```python
from build123d import *

# Parameters (mm, degrees)
F2_DEPTH     = 4
F0_R         = 11.5
F3_DEPTH     = 4
F4_T1_DEPTH  = 21.9483713996
F4_T3_DEPTH  = 22.3459559115
F4_T5_DEPTH  = 21.2495705846
F4_T7_DEPTH  = 22.5954800676
F4_T9_DEPTH  = 22.5954384353
F4_T11_DEPTH = 21.948545213


# Not quite as in the source:
# - a fillet or chamfer that OpenCascade refuses, or shapes differently, is made with other operations: its cross-section is extruded or revolved along the edge and cut away or added


with BuildPart() as f2:
    # F1 (on Top) → F2 (new body, symmetric)
    with BuildSketch(Plane.XY):
        with BuildLine():
            ThreePointArc((-24.434154737, 1.9297075548), (-16.0117202716, 5.9282775779), (-12.5894382026, 14.6008752276))
            ThreePointArc((-12.5894382026, 14.6008752276), (-12.8847624083, 17.3237447508), (-13.7570001617, 19.9199797418))
            Line((-13.7570001617, 19.9199797418), (-24.434154737, 1.9297075548))
        make_face()
        with BuildLine():
            ThreePointArc((-13.7570001617, 19.9199797418), (-12.8847624083, 17.3237447508), (-12.5894382026, 14.6008752276))
            ThreePointArc((-12.5894382026, 14.6008752276), (-16.0117202716, 5.9282775779), (-24.434154737, 1.9297075548))
            Line((-24.434154737, 1.9297075548), (-25.3981637022, 0.3054186533))
            Line((-25.3981637022, 0.3054186533), (-12.9635821636, -21.842745649))
            Line((-12.9635821636, -21.842745649), (-10.3728090059, -21.8739002812))
            ThreePointArc((-10.3728090059, -21.8739002812), (0.1527093266, -16.5024942777), (10.54601793, -22.1254538984))
            Line((10.54601793, -22.1254538984), (12.4345815386, -22.1481643023))
            Line((12.4345815386, -22.1481643023), (25.3981637022, -0.3054186533))
            Line((25.3981637022, -0.3054186533), (24.3123835544, 1.6285456733))
            ThreePointArc((24.3123835544, 1.6285456733), (13.9458157922, 8.2323089444), (13.7055148895, 20.5212337137))
            Line((13.7055148895, 20.5212337137), (12.9635821636, 21.842745649))
            Line((12.9635821636, 21.842745649), (-12.4345815386, 22.1481643023))
            Line((-12.4345815386, 22.1481643023), (-13.7570001617, 19.9199797418))
        make_face()
        with BuildLine():
            Line((-24.434154737, 1.9297075548), (-13.7570001617, 19.9199797418))
            ThreePointArc((-13.7570001617, 19.9199797418), (-36.2108110271, 21.0826663094), (-24.434154737, 1.9297075548))
        make_face()
        with BuildLine():
            Line((24.3123835544, 1.6285456733), (13.7055148895, 20.5212337137))
            ThreePointArc((13.7055148895, 20.5212337137), (13.9458157922, 8.2323089444), (24.3123835544, 1.6285456733))
        make_face()
        with BuildLine():
            ThreePointArc((38.29859269, 14.6009373546), (28.3341688507, 27.2487571734), (13.7055148895, 20.5212337137))
            Line((13.7055148895, 20.5212337137), (24.3123835544, 1.6285456733))
            ThreePointArc((24.3123835544, 1.6285456733), (34.136115438, 5.0628952085), (38.29859269, 14.6009373546))
        make_face()
        with BuildLine():
            Line((10.54601793, -22.1254538984), (-10.3728090059, -21.8739002812))
            ThreePointArc((-10.3728090059, -21.8739002812), (-3.8441725784, -41.3058041995), (12.7, -29.2015761288))
            ThreePointArc((12.7, -29.2015761288), (12.1495766945, -25.5032270182), (10.54601793, -22.1254538984))
        make_face()
        with BuildLine():
            ThreePointArc((10.54601793, -22.1254538984), (0.1527093266, -16.5024942777), (-10.3728090059, -21.8739002812))
            Line((-10.3728090059, -21.8739002812), (10.54601793, -22.1254538984))
        make_face()
    extrude(amount=F2_DEPTH, both=True)

    # F0 (on Top) → F3 (cut, symmetric)
    with BuildSketch(Plane.XY):
        with Locations((-25.4, 14.6646968374)):
            Circle(F0_R)
        with Locations((25.4, 14.6646968374)):
            Circle(F0_R)
        with Locations((0, -29.3293936748)):
            Circle(F0_R)
        Circle(F0_R)
    extrude(amount=F3_DEPTH, both=True, mode=Mode.SUBTRACT)

    # F4: fillet of radius 5.08 on 6 edges, made by hand

    # F4_s2 → F4_t1 (cut)
    with BuildSketch(Plane.XY.offset(-10.9741856998)):
        with BuildLine():
            ThreePointArc((10.54601793, -22.1254538984), (12.4510077343, -21.2841478503), (13.8583678275, -19.7491821865))
            Line((13.8583678275, -19.7491821865), (12.4345815386, -22.1481643023))
            Line((12.4345815386, -22.1481643023), (10.54601793, -22.1254538984))
        make_face()
    extrude(amount=F4_T1_DEPTH, mode=Mode.SUBTRACT)

    # F4_s4 → F4_t3 (cut)
    with BuildSketch(Plane.XY.offset(-11.1729779558)):
        with BuildLine():
            ThreePointArc((23.9337937954, -2.7727813782), (24.6265549669, -0.6154246052), (24.3123835544, 1.6285456733))
            Line((24.3123835544, 1.6285456733), (25.3981637022, -0.3054186533))
            Line((25.3981637022, -0.3054186533), (23.9337937954, -2.7727813782))
        make_face()
    extrude(amount=F4_T3_DEPTH, mode=Mode.SUBTRACT)

    # F4_s6 → F4_t5 (cut)
    with BuildSketch(Plane.XY.offset(-10.6247852923)):
        with BuildLine():
            ThreePointArc((10.3138596228, 21.8746091608), (12.1354983401, 21.5132129748), (13.7055148895, 20.5212337137))
            Line((13.7055148895, 20.5212337137), (12.9635821636, 21.842745649))
            Line((12.9635821636, 21.842745649), (10.3138596228, 21.8746091608))
        make_face()
    extrude(amount=F4_T5_DEPTH, mode=Mode.SUBTRACT)

    # F4_s8 → F4_t7 (cut)
    with BuildSketch(Plane.XY.offset(-11.2977400338)):
        with BuildLine():
            ThreePointArc((-13.7570001617, 19.9199797418), (-11.910066672, 21.54587795), (-9.5156965617, 22.1130640513))
            Line((-9.5156965617, 22.1130640513), (-12.4345815386, 22.1481643023))
            Line((-12.4345815386, 22.1481643023), (-13.7570001617, 19.9199797418))
        make_face()
    extrude(amount=F4_T7_DEPTH, mode=Mode.SUBTRACT)

    # F4_s10 → F4_t9 (cut)
    with BuildSketch(Plane.XY.offset(-11.2977192176)):
        with BuildLine():
            ThreePointArc((-14.3926228669, -19.2973742433), (-12.7042844419, -21.0873382025), (-10.3728090059, -21.8739002812))
            Line((-10.3728090059, -21.8739002812), (-12.9635821636, -21.842745649))
            Line((-12.9635821636, -21.842745649), (-14.3926228669, -19.2973742433))
        make_face()
    extrude(amount=F4_T9_DEPTH, mode=Mode.SUBTRACT)

    # F4_s12 → F4_t11 (cut)
    with BuildSketch(Plane.XY.offset(-10.9742726065)):
        with BuildLine():
            ThreePointArc((-24.0324603731, -2.1271378125), (-24.6581063385, -0.1407771898), (-24.434154737, 1.9297075548))
            Line((-24.434154737, 1.9297075548), (-25.3981637022, 0.3054186533))
            Line((-25.3981637022, 0.3054186533), (-24.0324603731, -2.1271378125))
        make_face()
    extrude(amount=F4_T11_DEPTH, mode=Mode.SUBTRACT)


solid = f2.part
```
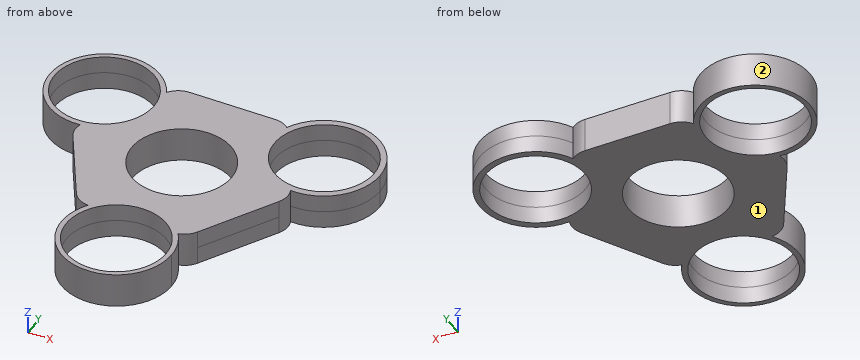
CAD build for the part. Positions are in the model's coordinates, mm. Face numbers are marked on the shaded views. Round coordinates to 2 decimals unless told otherwise and drop trailing zeros. Order: outer loops, then holes, each group sorted by start corner. A loop starts at its lowest first (then second) coordinate and runs counter-clockwise, first axis right, second up. Notation, with made-up numbers: (79, 60) - (115, 60) arc R22 cw to (115, 97) - close; hole circle Ø2 at (77, 52). An arc over 180 degrees is marked (long way). Use CSV: the item, a comma, the result in double quotes. Start each with the question number.
1) Wall check: L1, parallel to X at y = -29, z = -2.5; L2, parallel to Y at x = 25.4, z = -3.05; L3, parallel to Y at x = -25.4, z = 2.5. Give the ranges that are in metal, low to high. Write a range as [from, to].
2) Saw through at D-D (y = -31). List the corners of the cut face in (x, z).
3) Pin check, flat tips, straight feed: pin 1 Ø14 at (x, y) = (0, -29.33) entering from -Z; pin 2 Ø1.5 at (x, z) = (10, -1.5) entering from -Y. Stop position of each tip, or through.
4) Two-plate mould, pull along X, no slides. Class the marked faces 1 and 2: pulls with the +X half, pulls with the -X half, needs draft (parallel to the pull), parting line crosses it, or undercut.
5) Saw through at B-B (y = 16). List the corners of the cut face in (x, z), and give its area (3 significant figures).
6) Saw through at A-A (x = -4.5). List the corners of the cut face in (y, z).
7) Saw through at C-C (x = 19). List the corners of the cut face in (y, z), and give its area (3 significant figures).
Values follow:
1,L1,"x = [-12.7, -11.5], [11.5, 12.7]"
1,L2,"y = [1.59, 3.16], [26.16, 27.61]"
1,L3,"y = [1.9, 3.16], [26.16, 27.3]"
2,outline,"(-12.57, -4) - (-11.38, -4) - (-11.38, 4) - (-12.57, 4) - close; (11.38, -4) - (12.57, -4) - (12.57, 4) - (11.38, 4) - close"
3,pin 1,"passes through"
3,pin 2,"stops at y = -37.9"
4,face 1,"needs draft"
4,face 2,"undercut"
5,outline,"(-37.91, -4) - (-36.82, -4) - (-36.82, 4) - (-37.91, 4) - close; (-13.98, -4) - (13.98, -4) - (13.98, 4) - (-13.98, 4) - close; (36.82, -4) - (38.22, -4) - (38.22, 4) - (36.82, 4) - close"
5,area,"244 mm2"
6,outline,"(-41.08, -4) - (-39.91, -4) - (-39.91, 4) - (-41.08, 4) - close; (-18.75, -4) - (-10.58, -4) - (-10.58, 4) - (-18.75, 4) - close; (10.58, -4) - (22.05, -4) - (22.05, 4) - (10.58, 4) - close"
7,outline,"(-11.09, -4) - (5.11, -4) - (5.11, 4) - (-11.09, 4) - close; (24.22, -4) - (25.99, -4) - (25.99, 4) - (24.22, 4) - close"
7,area,"144 mm2"
